Design review of the part built by this model. Coordinates are the model's own, in mm. A direction names the side the tool comes from. Coordinates: 2 decimals unless noted, no trailing zeros. Write each loop counter-clockwise with the first axis right and the second up, starting at its lowest first coordinate (ties: lowest second). Pieces come first, ordered by that corner, then holes.
```python
from build123d import *

# Parameters (mm, degrees)
F0_R     = 50
F1_DEPTH = 3
F2_R     = 49
F2_R_2   = 42.5
F3_DEPTH = 5
F4_R     = 49
F4_R_2   = 48.25
F5_DEPTH = 7


with BuildPart() as f1:
    # F0 (on Top) → F1 (new body)
    with BuildSketch(Plane.XY):
        Circle(F0_R)
    extrude(amount=F1_DEPTH)

    # F2 (on face) → F3 (join)
    with BuildSketch(Plane.XY.offset(3)):
        Circle(F2_R)
        Circle(F2_R_2, mode=Mode.SUBTRACT)
    extrude(amount=F3_DEPTH)

    # F4 (on face) → F5 (join)
    with BuildSketch(Plane.XY.offset(8)):
        Circle(F4_R)
        Circle(F4_R_2, mode=Mode.SUBTRACT)
    extrude(amount=F5_DEPTH)


solid = f1.part
```
(1) For faces 1 (the flat face through (-1, 1, 3)), 2 (the flat face through (32.4, -36.1, 15)), list the 3-axis set-ups (+Z, -Z, +X, -X, +Y, -Y) from which the entire face can be reached by the end or side of a thin tool; tool diameter is ignored.
(2) Insertion check: pin 1 Ø8 at (x, z) = (-23.5, 8.5) entering from -Y; pin 2 Ø2 at (x, z) = (9.5, 8.5) entering from +Y; pin 3 Ø3 at (y, z) = (-2.5, 9.5) entering from +X. Each pin has a flat end and moves straight along its axis. Give the tip position at first contact, or say it passes through.
(3) Consider section C-C (z = 13). Give the boundary of the cut face in (x, y).
(4) Consider section D-D (y = 44). Give the boundary of the cut face in (x, z), plus the area to 3 significant figures.
(5) Mouldability with a two-part tool opening along X and no side actions: class faces 3 (the flat face through (-1, 1, 0)), 4 (the flat face through (0, -43, 8)), 5 (the cylindrical face through (47.69, 15.02, 1.48)) as +X half, -X half, draft (parallel to the pull), parting line (faces both ways), or undercut.
(6) Wall thickness on line 1 (Y direction, x = 0, z = 9.75); line 2 (Y direction, x = 0, z = 4.5); line 3 (X direction, y = -1, z = 7.25): over which ranges is each line inside the solid? List them lowest first.
(7) Consider section A-A (x = 0). Give the boundary of the cut face in (y, z), plus the area to 4 significant figures.
Results:
1. face 1: +Z
1. face 2: +Z, +X, -X, +Y, -Y
2. pin 1: stops at y = -44.95
2. pin 2: stops at y = 48.26
2. pin 3: stops at x = 48.99
3. outline: circle Ø98 at (0, 0); hole circle Ø96.5 at (0, 0)
4. outline: (-23.75, 0) - (23.75, 0) - (23.75, 3) - (21.56, 3) - (21.56, 15) - (19.8, 15) - (19.8, 8) - (-19.8, 8) - (-19.8, 15) - (-21.56, 15) - (-21.56, 3) - (-23.75, 3) - close
4. area: 383 mm2
5. face 3: draft
5. face 4: undercut
5. face 5: parting line
6. line 1: y = -49 to -48.25, 48.25 to 49
6. line 2: y = -49 to -42.5, 42.5 to 49
6. line 3: x = -48.99 to -42.49, 42.49 to 48.99
7. outline: (-50, 0) - (50, 0) - (50, 3) - (49, 3) - (49, 15) - (48.25, 15) - (48.25, 8) - (42.5, 8) - (42.5, 3) - (-42.5, 3) - (-42.5, 8) - (-48.25, 8) - (-48.25, 15) - (-49, 15) - (-49, 3) - (-50, 3) - close
7. area: 375.5 mm2
